Source: CAD feature listing. Evaluate the final solid. Frame: model axes, mm. A direction names the side the tool comes from. Give positions to 0.01 mm unless a question says otherwise; leave off trailing zeros. Loops run counter-clockwise (first coordinate to the right, second up) from the corner with the lowest first, then second, coordinate; pieces in that order, holes last. Notation, with made-up numbers: M 13,60.25 L 44,60.25 A17 ccw 44,87.25 Z; hole C -1,-16.5 d5. An arc over 180 degrees is marked long. Write item = value, one per line.
from build123d import *

# Parameters (mm, degrees)
SKETCH_3_R                  = 45
CUT_EXTRUDE_1_DEPTH         = 312.769145362
HOLE_WIZARD_4_D             = 4.5
HOLE_WIZARD_4_DEPTH         = 10
HOLE_WIZARD_4_CBORE_D       = 8
HOLE_WIZARD_4_CBORE_DEPTH   = 4.6
PATTERN_CIRCULAR_1_COUNT    = 10
MIRROR_1_COPY_1_D           = 4.5
MIRROR_1_COPY_1_DEPTH       = 10
MIRROR_1_COPY_1_CBORE_D     = 8
MIRROR_1_COPY_1_CBORE_DEPTH = 4.6
MIRROR_1_COPY_2_D           = 4.5
MIRROR_1_COPY_2_DEPTH       = 10
MIRROR_1_COPY_2_CBORE_D     = 8
MIRROR_1_COPY_2_CBORE_DEPTH = 4.6
MIRROR_1_COPY_3_D           = 4.5
MIRROR_1_COPY_3_DEPTH       = 10
MIRROR_1_COPY_3_CBORE_D     = 8
MIRROR_1_COPY_3_CBORE_DEPTH = 4.6
MIRROR_1_COPY_4_D           = 4.5
MIRROR_1_COPY_4_DEPTH       = 10
MIRROR_1_COPY_4_CBORE_D     = 8
MIRROR_1_COPY_4_CBORE_DEPTH = 4.6
MIRROR_1_COPY_5_D           = 4.5
MIRROR_1_COPY_5_DEPTH       = 10
MIRROR_1_COPY_5_CBORE_D     = 8
MIRROR_1_COPY_5_CBORE_DEPTH = 4.6
MIRROR_1_COPY_6_D           = 4.5
MIRROR_1_COPY_6_DEPTH       = 10
MIRROR_1_COPY_6_CBORE_D     = 8
MIRROR_1_COPY_6_CBORE_DEPTH = 4.6
MIRROR_1_COPY_7_D           = 4.5
MIRROR_1_COPY_7_DEPTH       = 10
MIRROR_1_COPY_7_CBORE_D     = 8
MIRROR_1_COPY_7_CBORE_DEPTH = 4.6
MIRROR_1_COPY_8_D           = 4.5
MIRROR_1_COPY_8_DEPTH       = 10
MIRROR_1_COPY_8_CBORE_D     = 8
MIRROR_1_COPY_8_CBORE_DEPTH = 4.6
MIRROR_1_COPY_9_D           = 4.5
MIRROR_1_COPY_9_DEPTH       = 10
MIRROR_1_COPY_9_CBORE_D     = 8
MIRROR_1_COPY_9_CBORE_DEPTH = 4.6


with BuildPart() as part:
    # 草图1 → 旋转1 (revolve)
    with BuildSketch(Plane.XY, mode=Mode.PRIVATE) as revolve_1_sk:
        Polygon((140, 50), (-140, 50), (-140, 60), (-150, 60), (-150, 0), (150, 0), (150, 60), (140, 60), align=None)
    revolve(revolve_1_sk.sketch.rotate(Axis((-150, 0, 0), (1, 0, 0)), 90), axis=Axis((-150, 0, 0), (1, 0, 0)))

    # 草图3 → 切除-拉伸1 (cut, through all)
    with BuildSketch(Plane(origin=(150, 0, 0), x_dir=(0, 0, -1), z_dir=(1, 0, 0))):
        Circle(SKETCH_3_R)
    extrude(amount=-CUT_EXTRUDE_1_DEPTH, mode=Mode.SUBTRACT)

    # 打孔尺寸(%根据)内六角圆柱头螺钉的类型4
    with Locations(Plane(origin=(-140, 0, 0), x_dir=(0, 0, -1), z_dir=(1, 0, 0))):
        with Locations((0, 55)):
            hole_wizard_4 = CounterBoreHole(HOLE_WIZARD_4_D / 2, HOLE_WIZARD_4_CBORE_D / 2, HOLE_WIZARD_4_CBORE_DEPTH, depth=HOLE_WIZARD_4_DEPTH)

    # 阵列(圆周)1: 打孔尺寸(%根据)内六角圆柱头螺钉的类型4 ×10 about axis
    pattern_circular_1_axis = Axis((0, 0, 0), (1, 0, 0))
    for i in range(1, PATTERN_CIRCULAR_1_COUNT):
        add(hole_wizard_4.rotate(pattern_circular_1_axis, i * 360 / PATTERN_CIRCULAR_1_COUNT), mode=Mode.SUBTRACT)

    # 镜向1: 打孔尺寸(%根据)内六角圆柱头螺钉的类型4 across plane
    add(hole_wizard_4.mirror(Plane(origin=(0, 0, 0), x_dir=(0, 0, 1), z_dir=(1, 0, 0))), mode=Mode.SUBTRACT)

    # 镜向1 copy 1
    with Locations(Plane(origin=(140, 0, 0), x_dir=(0, 0.5877852522924731, -0.8090169943749475), z_dir=(-1, 0, 0))):
        with Locations((0, -55)):
            CounterBoreHole(MIRROR_1_COPY_1_D / 2, MIRROR_1_COPY_1_CBORE_D / 2, MIRROR_1_COPY_1_CBORE_DEPTH, depth=MIRROR_1_COPY_1_DEPTH)

    # 镜向1 copy 2
    with Locations(Plane(origin=(140, 0, 0), x_dir=(0, 0.9510565162951535, -0.30901699437494745), z_dir=(-1, 0, 0))):
        with Locations((0, -55)):
            CounterBoreHole(MIRROR_1_COPY_2_D / 2, MIRROR_1_COPY_2_CBORE_D / 2, MIRROR_1_COPY_2_CBORE_DEPTH, depth=MIRROR_1_COPY_2_DEPTH)

    # 镜向1 copy 3
    with Locations(Plane(origin=(140, 0, 0), x_dir=(0, 0.9510565162951536, 0.30901699437494734), z_dir=(-1, 0, 0))):
        with Locations((0, -55)):
            CounterBoreHole(MIRROR_1_COPY_3_D / 2, MIRROR_1_COPY_3_CBORE_D / 2, MIRROR_1_COPY_3_CBORE_DEPTH, depth=MIRROR_1_COPY_3_DEPTH)

    # 镜向1 copy 4
    with Locations(Plane(origin=(140, 0, 0), x_dir=(0, 0.5877852522924732, 0.8090169943749473), z_dir=(-1, 0, 0))):
        with Locations((0, -55)):
            CounterBoreHole(MIRROR_1_COPY_4_D / 2, MIRROR_1_COPY_4_CBORE_D / 2, MIRROR_1_COPY_4_CBORE_DEPTH, depth=MIRROR_1_COPY_4_DEPTH)

    # 镜向1 copy 5
    with Locations(Plane.ZY.offset(-140)):
        with Locations((0, -55)):
            CounterBoreHole(MIRROR_1_COPY_5_D / 2, MIRROR_1_COPY_5_CBORE_D / 2, MIRROR_1_COPY_5_CBORE_DEPTH, depth=MIRROR_1_COPY_5_DEPTH)

    # 镜向1 copy 6
    with Locations(Plane(origin=(140, 0, 0), x_dir=(0, -0.587785252292473, 0.8090169943749476), z_dir=(-1, 0, 0))):
        with Locations((0, -55)):
            CounterBoreHole(MIRROR_1_COPY_6_D / 2, MIRROR_1_COPY_6_CBORE_D / 2, MIRROR_1_COPY_6_CBORE_DEPTH, depth=MIRROR_1_COPY_6_DEPTH)

    # 镜向1 copy 7
    with Locations(Plane(origin=(140, 0, 0), x_dir=(0, -0.9510565162951535, 0.30901699437494756), z_dir=(-1, 0, 0))):
        with Locations((0, -55)):
            CounterBoreHole(MIRROR_1_COPY_7_D / 2, MIRROR_1_COPY_7_CBORE_D / 2, MIRROR_1_COPY_7_CBORE_DEPTH, depth=MIRROR_1_COPY_7_DEPTH)

    # 镜向1 copy 8
    with Locations(Plane(origin=(140, 0, 0), x_dir=(0, -0.9510565162951536, -0.30901699437494723), z_dir=(-1, 0, 0))):
        with Locations((0, -55)):
            CounterBoreHole(MIRROR_1_COPY_8_D / 2, MIRROR_1_COPY_8_CBORE_D / 2, MIRROR_1_COPY_8_CBORE_DEPTH, depth=MIRROR_1_COPY_8_DEPTH)

    # 镜向1 copy 9
    with Locations(Plane(origin=(140, 0, 0), x_dir=(0, -0.5877852522924734, -0.8090169943749473), z_dir=(-1, 0, 0))):
        with Locations((0, -55)):
            CounterBoreHole(MIRROR_1_COPY_9_D / 2, MIRROR_1_COPY_9_CBORE_D / 2, MIRROR_1_COPY_9_CBORE_DEPTH, depth=MIRROR_1_COPY_9_DEPTH)


solid = part.part
1. Cut plane B-B, the plane z = 7.5. Return the cut outline in (x, y).
Derived:
outline = M -150,-59.53 L -140,-59.53 L -140,-49.43 L 140,-49.43 L 140,-59.53 L 150,-59.53 L 150,-44.37 L -150,-44.37 Z; M -150,44.37 L 150,44.37 L 150,59.53 L 140,59.53 L 140,49.43 L -140,49.43 L -140,59.53 L -150,59.53 Z
2. First-contact query: pin 1 Ø2.5 at (y, z) = (-44.5, 32.33) entering from -X; pin 2 Ø1 at (x, z) = (56, 29) entering from -Y; pin 3 Ø2 at (x, y) = (-92.5, -10.5) entering from -Z; pin 4 Ø10 at (x, z) = (61.5, -38.5) entering from -Y. Flat tips, straight axial feed; report the tip coordinate or a pass-through.
Derived:
pin_1 = through
pin_2 = -41.08
pin_3 = -49.09
pin_4 = -37.12
3. Material intervals for probe 1 along Y at (x, z) = (-145.75, 0); probe 2 along X at (y, z) = (-51.5, 8.5); probe 3 along Y at (x, z) = (-126, 0.5), sorted ascending. Write a range as from..to.
Derived:
probe_1 = -60..-57.25, -52.75..-45, 45..52.75, 57.25..60
probe_2 = -150..-140, 140..150
probe_3 = -50..-45, 45..50
4. Reachability of faces 1 (the flat face through (-144.6, -18, -50)), 2 (the flat face through (-150, 9, -45)) from +Z, -Z, +X, -X, +Y, -Y: full face, straight path, thin tool, end or side. Return the list, or none.
Derived:
face_1 = none
face_2 = +Z, -Z, -X, +Y, -Y
5. Pull-direction query (Y, two-part tool) for faces 3 (the cylindrical face through (-1.96, -15.02, 47.69)), 4 (the flat face through (144.6, -15.9, 54.5)), 5 (the flat face through (150, 9, 45)); classes: +Y half, -Y half, draft (parallel to the pull), parting line (faces both ways), or undercut.
Derived:
face_3 = parting line
face_4 = undercut
face_5 = draft
6. Cut plane A-A, the plane y = -29.5. Return the cut outline in (x, z).
Derived:
outline = M -150,-52.25 L -140,-52.25 L -140,-40.37 L 140,-40.37 L 140,-52.25 L 150,-52.25 L 150,-33.98 L -150,-33.98 Z; M -150,33.98 L 150,33.98 L 150,52.25 L 140,52.25 L 140,40.37 L -140,40.37 L -140,52.25 L -150,52.25 Z
7. Cut plane C-C, the plane x = 37. Return the cut outline in (y, z), then the cut area to 3 significant figures.
Derived:
outline = C 0,0 d100; hole C 0,0 d90
area = 1,490 mm²
